Autodesk Inventor part; units mm, degrees
ref_plane "side_2a_XY" through (61.137, 0, 0) normal (0, 0, 1) x (1, 0, 0)
ref_plane "side_2a_YZ" through (61.137, 0, 0) normal (1, 0, 0) x (0, 1, 0)
ref_plane "side_2a_ZX" through (61.137, 0, 0) normal (0, 1, 0) x (0, 0, 1)
sketch "Skizze_1" plane through (0, 0, 0) normal (0, 1, 0) x (-1, 0, 0)
  line L0 (73.8629, -73.8629) -> (0, 0)
  line L1 (0, 0) -> (-86.1371, 0)
  line L2 (-86.1371, 0) -> (-86.1371, -27)
  line L3 (-86.1371, -27) -> (46.8629, -160)
  line L4 (46.8629, -160) -> (73.8629, -160)
  line L5 (73.8629, -160) -> (73.8629, -73.8629)
  circle A0 centre (27.8629, -96) radius 8.7
extrude "Extrusion1" add sketch "Skizze_1" along normal mid plane 25
sketch "Skizze_2" plane through (0, 0, 0) normal (0, 1, 0) x (1, 0, 0)
  line L0 (72.1371, 0) -> (75.5513, -3.4142)
  arc A0 (75.5513, -3.4142) -> (76.9655, -4) centre (76.9655, -2) ccw
  line L1 (76.9655, -4) -> (84.1371, -4)
  arc A1 (84.1371, -4) -> (86.1371, -2) centre (84.1371, -2) ccw
  line L2 (86.1371, -2) -> (86.1371, 0)
  line L3 (86.1371, 0) -> (72.1371, 0)
extrude "Extrusion2" add sketch "Skizze_2" along normal mid plane 8
sketch "Skizze_3" plane through (0, 0, 0) normal (0, 1, 0) x (1, 0, 0)
  line L0 (0, 0) -> (3.4142, -3.4142)
  arc A0 (3.4142, -3.4142) -> (4.8284, -4) centre (4.8284, -2) ccw
  line L1 (4.8284, -4) -> (44.8087, -4)
  arc A1 (44.8087, -4) -> (46.2229, -3.4142) centre (44.8087, -2) ccw
  line L2 (46.2229, -3.4142) -> (49.6371, 0)
  line L3 (49.6371, 0) -> (0, 0)
extrude "Extrusion3" add sketch "Skizze_3" along normal mid plane 8
sketch "Skizze_4" plane through (0, 0, 0) normal (0, 1, 0) x (1, 0, 0)
  arc A0 (-77.8629, 150.8284) -> (-77.2771, 149.4142) centre (-75.8629, 150.8284) ccw
  line L0 (-77.2771, 149.4142) -> (-73.8629, 146)
  line L1 (-73.8629, 146) -> (-73.8629, 160)
  line L2 (-73.8629, 160) -> (-75.8629, 160)
  arc A1 (-75.8629, 160) -> (-77.8629, 158) centre (-75.8629, 158) ccw
  line L3 (-77.8629, 158) -> (-77.8629, 150.8284)
extrude "Extrusion4" add sketch "Skizze_4" along normal mid plane 8
sketch "Skizze_5" plane through (0, 0, 0) normal (0, 1, 0) x (1, 0, 0)
  line L0 (-77.8629, 118.6716) -> (-77.8629, 78.6913)
  arc A0 (-77.8629, 78.6913) -> (-77.2771, 77.2771) centre (-75.8629, 78.6913) ccw
  line L1 (-77.2771, 77.2771) -> (-73.8629, 73.8629)
  line L2 (-73.8629, 73.8629) -> (-73.8629, 123.5)
  line L3 (-73.8629, 123.5) -> (-77.2771, 120.0858)
  arc A1 (-77.2771, 120.0858) -> (-77.8629, 118.6716) centre (-75.8629, 118.6716) ccw
extrude "Extrusion5" add sketch "Skizze_5" along normal mid plane 8
sketch "Sketch6" plane through (0, -12.5, 0) normal (0, 0, 1) x (1, 0, 0)
  point P0 (61.1371, 12.5)
hole "Drilling 1" at (61.1371, 0, 0) direction (0, 0, -1) diameter 9 depth 92.3404
sketch "Skizze_7" plane through (0, 0, 0) normal (0, 1, 0) x (1, 0, 0)
  line L0 (50, 135) -> (-50, 135)
  line L1 (-73.8629, 135) -> (-73.8629, 139.5)
  line L2 (-73.8629, 139.5) -> (0, 139.5)
  line L3 (0, 139.5) -> (0, 135)
  line L4 (0, 135) -> (-73.8629, 135)
revolve "Revolution1" cut sketch "Skizze_7" angle 360 about axis through (50, 0, -135) along (1, 0, 0)
sketch "Skizze_8" plane through (0, 0, 0) normal (0, 1, 0) x (1, 0, 0)
  line L0 (-46.1238, 53.1949) -> (-36.2244, 43.2954)
  line L1 (-36.2244, 43.2954) -> (0.0798, 76.9104)
  arc A0 (3.0475, 73.9428) -> (0.0798, 76.9104) centre (1.5066, 75.3695) ccw
  line L2 (3.0475, 73.9428) -> (-30.5675, 37.6386)
  line L3 (-30.5675, 37.6386) -> (-20.668, 27.7391)
  line L4 (-20.668, 27.7391) -> (12.566, 58.1447)
  line L5 (12.566, 58.1447) -> (42.9716, 70.1655)
  line L6 (42.9716, 70.1655) -> (-3.6974, 116.8345)
  line L7 (-3.6974, 116.8345) -> (-15.7183, 86.4289)
  line L8 (-15.7183, 86.4289) -> (-46.1238, 53.1949)
extrude "Extrusion6" cut sketch "Skizze_8" along normal mid plane 10
sketch "Sketch9" plane through (0, 12.5, 0) normal (0, 1, 0) x (1, 0, 0)
  point P0 (22.1, 46)
hole "Drilling 3" at (22.1, 12.5, -46) direction (0, -1, 0) diameter 11.835 depth 25 countersink diameter 14 countersink angle 90
sketch "Skizze_10" plane through (0, 0, 0) normal (0, 1, 0) x (1, 0, 0)
  line L0 (-3.5355, 8.5355) -> (0, 5)
  line L1 (0, 5) -> (37.9741, 5)
  line L2 (37.9741, 5) -> (46.8927, 13.9185)
  line L3 (46.8927, 13.9185) -> (69.5201, 13.9185)
  line L4 (69.5201, 13.9185) -> (84.3693, 28.7678)
  line L5 (84.3693, 28.7678) -> (45.4465, 67.6906)
  line L6 (45.4465, 67.6906) -> (24.3701, 36.4411)
  line L7 (24.3701, 36.4411) -> (-3.5355, 8.5355)
extrude "Extrusion7" cut sketch "Skizze_10" along normal mid plane 10
sketch "Skizze_11" plane through (0, 0, 0) normal (0, 1, 0) x (1, 0, 0)
  line L0 (-68.8629, 73.8629) -> (-65.3274, 70.3274)
  line L1 (-65.3274, 70.3274) -> (-39.1198, 102.7044)
  line L2 (-39.1198, 102.7044) -> (-6.1723, 119.3094)
  line L3 (-6.1723, 119.3094) -> (-45.0951, 158.2322)
  line L4 (-45.0951, 158.2322) -> (-59.9444, 143.383)
  line L5 (-59.9444, 143.383) -> (-59.9444, 120.7556)
  line L6 (-59.9444, 120.7556) -> (-68.8629, 111.837)
  line L7 (-68.8629, 111.837) -> (-68.8629, 73.8629)
extrude "Extrusion8" cut sketch "Skizze_11" along normal mid plane 10
ref_plane "side_2a_XY" through (61.137, 0, 0) normal (0, 0, 1) x (1, 0, 0)
ref_plane "side_2a_YZ" through (61.137, 0, 0) normal (1, 0, 0) x (0, 1, 0)
ref_plane "side_2a_ZX" through (61.137, 0, 0) normal (0, 1, 0) x (0, 0, 1)
ref_plane "side_2b_XY" through (61.137, 0, -13.919) normal (0, 0, -1) x (1, 0, 0)
ref_plane "side_2b_YZ" through (61.137, 0, -13.919) normal (1, 0, 0) x (0, -1, 0)
ref_plane "side_2b_ZX" through (61.137, 0, -13.919) normal (0, -1, 0) x (0, 0, -1)
ref_plane "side_5a_XY" through (-73.863, 0, -135) normal (-1, 0, 0) x (0, 0, -1)
ref_plane "side_5a_YZ" through (-73.863, 0, -135) normal (0, 0, -1) x (0, -1, 0)
ref_plane "side_5a_ZX" through (-73.863, 0, -135) normal (0, -1, 0) x (-1, 0, 0)
ref_plane "side_5b_XY" through (-59.944, 0, -135) normal (1, 0, 0) x (0, 0, -1)
ref_plane "side_5b_YZ" through (-59.944, 0, -135) normal (0, 0, -1) x (0, 1, 0)
ref_plane "side_5b_ZX" through (-59.944, 0, -135) normal (0, 1, 0) x (1, 0, 0)
ref_plane "side_1a_XY" through (22.137, 12, -46) normal (0, 1, 0) x (1, 0, 0)
ref_plane "side_1a_YZ" through (22.137, 12, -46) normal (1, 0, 0) x (0, 0, -1)
ref_plane "side_1a_ZX" through (22.137, 12, -46) normal (0, 0, -1) x (0, 1, 0)
ref_plane "side_1b_XY" through (-27.863, 12, -96) normal (0, 1, 0) x (1, 0, 0)
ref_plane "side_1b_YZ" through (-27.863, 12, -96) normal (1, 0, 0) x (0, 0, -1)
ref_plane "side_1b_ZX" through (-27.863, 12, -96) normal (0, 0, -1) x (0, 1, 0)
ref_plane "side_6a_XY" through (22.137, -12, -46) normal (0, -1, 0) x (1, 0, 0)
ref_plane "side_6a_YZ" through (22.137, -12, -46) normal (1, 0, 0) x (0, 0, 1)
ref_plane "side_6a_ZX" through (22.137, -12, -46) normal (0, 0, 1) x (0, -1, 0)
ref_plane "side_6b_XY" through (-27.863, -12, -96) normal (0, -1, 0) x (1, 0, 0)
ref_plane "side_6b_YZ" through (-27.863, -12, -96) normal (1, 0, 0) x (0, 0, 1)
ref_plane "side_6b_ZX" through (-27.863, -12, -96) normal (0, 0, 1) x (0, -1, 0)
properties part number "May Tec 1.47.225160.2_Floor mounting plate_schwarz-Pulverbeschichtet"
Geometry: final body of the model. Coordinates: model frame, mm. A direction names the side the tool comes from. Give positions to 0.01 mm unless a question says otherwise; leave off trailing zeros. Write each loop counter-clockwise with the first axis right and the second up, starting at its lowest first coordinate (ties: lowest second). Pieces come first, ordered by that corner, then holes. Notation, with made-up numbers: (15.25, -16) - (19.25, -16) arc R23 ccw to (19.25, 5) - close; hole circle Ø5 at (54, 9). An arc over 180 degrees is marked (long way). Return JSON: item names as keys, results as strings. Group by question number.
1) Section D-D on y = 0. State how many separate pieces and enclosed holes the cut face has, plus the area to 3 significant figures.
2) First-contact query: P1, Ø12, axis at x = -33.5, z = -102.5, coming from the -Y side; P2, Ø4, axis at x = -1.5, y = -5, coming from the +Z side; P3, Ø3, axis at y = -2.5, z = -124, coming from the -X side; P4, Ø11, axis at y = 2.5, z = -127.5, coming from the +X side. Flat tips, straight axial feed; report the tip coordinate or a pass-through.
3) Line query: line 1 (Y direction, x = -37, z = -122); line 2 (X direction, y = 2.25, z = -46); line 3 (Y direction, x = -65, z = -135). Output: solid intervals per line, ascending.
4) Section B-B on x = 22.1. Return the cut outline in (y, z), plus the area to 3 significant figures.
5) Section A-A on z = -90.5. Return the cut outline in (x, y).
6) Mould query, pull axis Y, two halves, no side actions, for faces 1 (the flat face through (25, 0, 4)), 2 (the flat face through (-4.28, -0.07, -42.73)), 3 (the flat face through (-76, 4, -155)). Classes: released by +Y, released by -Y, zero draft, split by the parting line, or undercut.
7) Section C-C on z = -46. Return the cut outline in (x, y).
8) Set-up query: faces 4 (the flat face through (-76, -4, -155)), 5 (the flat face through (27.556, -0.07, -64.071)), 6 (the flat face through (24, 4, 2)), 7 (the flat face through (-13.525, -0.07, -56.045)). Return all of +Z, -Z, +X, -X, +Y, -Y with unobstructed straight access to the full face (end or side cutting, diameter ignored); none if empty.
Filled in:
{
 "1": {"separate pieces": "3", "enclosed holes": "2", "area": "5,730 mm^2"},
 "2": {"P1": "stops at y = -12.5", "P2": "stops at z = 0.23", "P3": "stops at x = -74.86", "P4": "stops at x = -9.46"},
 "3": {"line 1": "y = -12.5 to -5, 5 to 12.5", "line 2": "x = -46 to -38.93, -33.3 to -22.83, -0.71 to 16.18, 28.02 to 30.82", "line 3": "y = -12.5 to -4.5, 4.5 to 12.5"},
 "4": {"outline": "(-12.5, -91.04) - (-5, -91.04) - (-5, -61.91) - (5, -61.91) - (5, -91.04) - (12.5, -91.04) - (12.5, -53) - (11.42, -51.92) - (-12.5, -51.92) - close; (-12.5, -40.08) - (11.42, -40.08) - (12.5, -39) - (12.5, 0) - (4, 0) - (4, 4) - (-4, 4) - (-4, 0) - (-12.5, 0) - close; hole (-5, -34.17) - (5, -34.17) - (5, -5) - (-5, -5) - close", "area": "1,430 mm^2"},
 "5": {"outline": "(-77.86, -4) - (-73.86, -4) - (-73.86, -12.5) - (-34.6, -12.5) - (-34.6, 12.5) - (-73.86, 12.5) - (-73.86, 4) - (-77.86, 4) - close; (-21.12, -12.5) - (22.64, -12.5) - (22.64, -5) - (-14.11, -5) - (-14.11, 5) - (22.64, 5) - (22.64, 12.5) - (-21.12, 12.5) - close; hole (-68.86, -5) - (-49, -5) - (-49, 5) - (-68.86, 5) - close"},
 "6": {"face 1": "zero draft", "face 2": "undercut", "face 3": "released by +Y"},
 "7": {"outline": "(-46, -12.5) - (16.18, -12.5) - (16.18, 11.42) - (15.1, 12.5) - (-46, 12.5) - close; (28.02, -12.5) - (67.14, -12.5) - (67.14, -5) - (30.82, -5) - (30.82, 5) - (67.14, 5) - (67.14, 12.5) - (29.1, 12.5) - (28.02, 11.42) - close; hole (-38.93, -5) - (-33.3, -5) - (-33.3, 5) - (-38.93, 5) - close; hole (-22.83, -5) - (-0.71, -5) - (-0.71, 5) - (-22.83, 5) - close"},
 "8": {"face 4": "+Z, -Z, -X, -Y", "face 5": "-Z", "face 6": "+Z, +X, -X, +Y", "face 7": "none"}
}
